CAD build for the part. Positions are in the model's coordinates, mm. A direction names the side the tool comes from. Round coordinates to 2 decimals unless told otherwise and drop trailing zeros. Loops run counter-clockwise (first coordinate to the right, second up) from the corner with the lowest first, then second, coordinate; pieces in that order, holes last. Notation, with made-up numbers: M 84,50.5 L 94,50.5 A34 ccw 94,87.5 Z; hole C 30,43 d8. An arc over 180 degrees is marked long. Use a Markdown table: item, result. Add a question column.
(1) Flat gauge pins, fed straight in: P1, Ø2.5, axis at x = -1.26, y = -17.96, coming from the -Z side; P2, Ø2, axis at y = -1, z = -43, coming from the +X side; P3, Ø1.2, axis at x = -2, z = -41.5, coming from the +Y side. Where does each tip first touch, or does it go through?
(2) Two-plate mould, pull along X, no slides. Class faces 1 (the face through (9.357, -14.297, -41.972)), 2 (the face through (4.71, -20.41, -41.97)), 3 (the face through (-11.39, -17.61, -41.97)): released by +X, released by -X, zero draft, split by the parting line, or undercut.
(3) Band-saw the part on C-C, the plane x = 18. Write the cut outline in (y, z), and give its area (3 significant figures).
(4) Wall check: L1, parallel to Y at x = -12, z = -41.95; L2, parallel to Y at x = -2.5, z = -41.7; L3, parallel to X at y = 16.5, z = -40.55. Give the ranges that are in metal, low to high.
(5) Band-saw the part on D-D, the plane y = 2. Write the cut outline in (x, z).
(6) Band-saw the part on A-A, the plane x = 1.5. Write the cut outline in (y, z), and give its area (3 significant figures).
(7) Band-saw the part on B-B, the plane y = 15. Write the cut outline in (x, z).
(8) Which spindle directions (+Z, -Z, +X, -X, +Y, -Y) get a long thin tool onto all of the face, cutting with end or side? Do faces 4 (the face through (4.65, 25.58, -41.97)), 5 (the face through (-9.4, -9.43, -42.03)). Say none if no direction does.
from build123d import *

# Parameters (mm, degrees)
PAD009_DEPTH          = 4
POLARPATTERN003_COUNT = 4
SKETCH018_R           = 1.65
HOLE003_DEPTH         = 25
POCKET006_DEPTH       = 149.7520027338
POLARPATTERN001_COUNT = 4
SKETCH024_W           = 20
SKETCH024_H           = 20
POCKET007_DEPTH       = 4.001
FILLET_R              = 2


with BuildPart() as part:
    # Sketch → Pad009 (new body)
    with BuildSketch(Plane.XY):
        with BuildLine():
            ThreePointArc((18.9209111487, -11.036007045), (25.6050015783, -4.5148526193), (21.5543772962, 3.8991216402))
            ThreePointArc((19.510343337, 5.7262546507), (20.4266011455, 4.694374188), (21.5543772962, 3.8991216402))
            Line((19.510343337, 5.7262546507), (15.7820965007, 11.0507429386))
            Line((0, 0), (15.7820965007, 11.0507429386))
            Line((0, 0), (11.0507429386, -15.7820965007))
            Line((11.0507429386, -15.7820965007), (16.3752312264, -12.0538496644))
            ThreePointArc((18.9209111487, -11.036007045), (17.5891558316, -11.3975778351), (16.3752312264, -12.0538496644))
        make_face()
    pad009 = extrude(amount=-PAD009_DEPTH)

    # PolarPattern003: Pad009 ×4 about axis
    polarpattern003_axis = Axis((0, 0, 0), (0, 0, 1))
    for i in range(1, POLARPATTERN003_COUNT):
        add(pad009.rotate(polarpattern003_axis, i * 360 / POLARPATTERN003_COUNT))

    # Sketch018 → Hole003 (cut)
    with BuildSketch(Plane.XY.offset(8)):
        with Locations((1.2556165274, 17.9561529047)):
            Circle(SKETCH018_R)
        with Locations((-1.2556165274, -17.9561529047)):
            Circle(SKETCH018_R)
        with Locations((-17.9561529047, 1.2556165274)):
            Circle(SKETCH018_R)
        with Locations((17.9561529047, -1.2556165274)):
            Circle(SKETCH018_R)
    extrude(amount=-HOLE003_DEPTH, mode=Mode.SUBTRACT)

    # Sketch021 → Pocket006 (cut, through all)
    with BuildSketch(Plane.XY):
        Polygon((11.2159688683, 12.0143126733), (12.0351209126, 12.5878891096), (16.6237324034, 6.0346727553), (15.8045803591, 5.461096319), align=None)
    pocket006 = extrude(amount=-POCKET006_DEPTH, mode=Mode.SUBTRACT)

    # PolarPattern001: Pocket006 ×4 about axis
    polarpattern001_axis = Axis((0, 0, 0), (0, 0, 1))
    for i in range(1, POLARPATTERN001_COUNT):
        add(pocket006.rotate(polarpattern001_axis, i * 360 / POLARPATTERN001_COUNT), mode=Mode.SUBTRACT)

    # Sketch024 → Pocket007 (cut, through all)
    with BuildSketch(Plane.XY):
        Rectangle(SKETCH024_W, SKETCH024_H)
    extrude(amount=-POCKET007_DEPTH, mode=Mode.SUBTRACT)

    # Fillet
    fillet_edges = [part.edges().sort_by_distance(p)[0] for p in [
        (10, -10, -2),
        (-10, -10, -2),
        (-10, 10, -2),
        (10, 10, -2),
    ]]
    fillet(fillet_edges, radius=FILLET_R)


with BuildPart() as part_1:
    # Body004024 placement: moved
    add(part.part.moved(Location((0, 0, -40))))


solid = part_1.part
Return value:
| question | item | result |
|---|---|---|
| 1 | P1 | through |
| 1 | P2 | x = 25.65 |
| 1 | P3 | y = 24.32 |
| 2 | face 1 | undercut |
| 2 | face 2 | released by +X |
| 2 | face 3 | released by -X |
| 3 | outline | M -11.25,-44 L -2.91,-44 L -2.91,-40 L -11.25,-40 Z; M 0.39,-44 L 7.88,-44 L 7.88,-40 L 0.39,-40 Z |
| 3 | area | 63.3 mm^2 |
| 4 | L1 | -16.45 to -12.56, -10.89 to 11.23, 12.45 to 15.12 |
| 4 | L2 | -25.7 to -19.04, -16.87 to -10, 10 to 23.41 |
| 4 | L3 | -10.03 to -6.21, -5.95 to 0.48, 2.03 to 11.97 |
| 5 | outline | M -25.65,-44 L -19.43,-44 L -19.43,-40 L -25.65,-40 Z; M -16.48,-44 L -10,-44 L -10,-40 L -16.48,-40 Z; M 10,-44 L 23.87,-44 L 23.87,-40 L 10,-40 Z |
| 6 | outline | M -24.25,-44 L -10,-44 L -10,-40 L -24.25,-40 Z; M 10,-44 L 16.32,-44 L 16.32,-40 L 10,-40 Z; M 19.59,-44 L 25.56,-44 L 25.56,-40 L 19.59,-40 Z |
| 6 | area | 106 mm^2 |
| 7 | outline | M -12.17,-44 L -8.35,-44 L -8.35,-40 L -12.17,-40 Z; M -6.61,-44 L 13.02,-44 L 13.02,-40 L -6.61,-40 Z |
| 8 | face 4 | +Z, -Z, +Y |
| 8 | face 5 | +Z, -Z |
